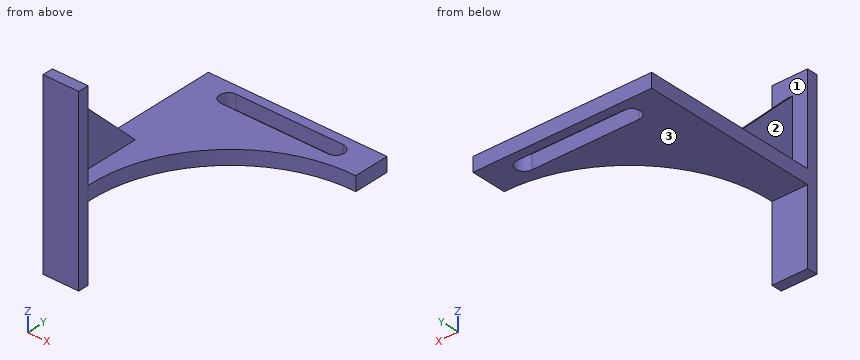
from build123d import *

# Parameters (mm, degrees)
SKETCH1_W           = 50
SKETCH1_H           = 15
BOSS_EXTRUDE1_DEPTH = 250
BOSS_EXTRUDE3_START = -135
BOSS_EXTRUDE3_DEPTH = 10
BOSS_EXTRUDE4_DEPTH = 3.75
CUT_EXTRUDE1_DEPTH  = 365.082751583


with BuildPart() as part:
    # Sketch1 → Boss-Extrude1 (new body)
    with BuildSketch(Plane.XY):
        Rectangle(SKETCH1_W, SKETCH1_H)
    extrude(amount=-BOSS_EXTRUDE1_DEPTH)

    # Sketch2 → Boss-Extrude3 (add, symmetric)
    with BuildSketch(Plane.XY.offset(BOSS_EXTRUDE3_START)):
        with BuildLine():
            Line((-25, 7.5), (-25, 257.5))
            Line((-25, 257.5), (225, 257.5))
            Line((225, 257.5), (225, 207.5))
            ThreePointArc((225, 207.5), (82.048365399, 150.451634601), (25, 7.5))
            Line((25, 7.5), (-25, 7.5))
        make_face()
    extrude(amount=BOSS_EXTRUDE3_DEPTH, both=True)

    # Sketch4 → Boss-Extrude4 (add, symmetric)
    with BuildSketch(Plane(origin=(0, 0, 0), x_dir=(0, 0, -1), z_dir=(1, 0, 0))):
        Polygon((25, 7.5), (125, 107.5), (125, 7.5), align=None)
    extrude(amount=BOSS_EXTRUDE4_DEPTH, both=True)

    # Sketch5 → Cut-Extrude1 (cut, through all)
    with BuildSketch(Plane.XY.offset(-125)):
        with BuildLine():
            Line((25, 244.5), (175, 244.5))
            ThreePointArc((175, 244.5), (187, 232.5), (175, 220.5))
            Line((175, 220.5), (25, 220.5))
            ThreePointArc((25, 220.5), (13, 232.5), (25, 244.5))
        make_face()
    extrude(amount=-CUT_EXTRUDE1_DEPTH, mode=Mode.SUBTRACT)


solid = part.part
Can you work these out from the model? Positions are in its coordinate system, mm. Face numbers are marked on the shaded views. A direction names the side the tool comes from. Give positions to 0.01 mm unless a question says otherwise; leave off trailing zeros. Write each loop counter-clockwise with the first axis right and the second up, starting at its lowest first coordinate (ties: lowest second). Pieces come first, ordered by that corner, then holes. Notation, with made-up numbers: (15, 62) -> (71, 62) arc R27 ccw to (71, 78) -> close; hole circle Ø9 at (-37, 45). An arc over 180 degrees is marked (long way). Answer as a JSON object with one key per item and string values. Group by question number.
Item 1: Suppose I cut it at D-D (y = 23). Please give me the cut outline in (x, z), plus the area to 3 significant figures.
Item 2: Please list where these lines run through material, in increasing order: line 1 (X direction, y = 26.5, z = -46); line 2 (Z direction, x = 130.5, y = 219.5); line 3 (Y direction, x = 20, z = -50.5). Write a range as [from, to].
Item 3: For the marked faces 1, 2 and 3, which set-ups out of +Z, -Z, +X, -X, +Y, -Y let a thin tool reach every point of the face, with its end or its side?
Item 4: Suppose I cut it at B-B (x = 83.5). Please give me the cut outline in (y, z).
Item 5: Suppose I cut it at C-C (z = -113.5). Please give me the cut outline in (x, y), plus the area to 3 significant figures.
Item 6: I'm going to push flat-ended pins straight in: P1, Ø4, axis at y = 26, z = -100.5, coming from the -X side; P2, Ø4, axis at x = 96.5, y = 201.5, coming from the -Z side; P3, Ø25, axis at x = -2, z = -213.5, coming from the +Y side. Where does each tip first touch, or does it pass through?
Item 7: Suppose I cut it at A-A (y = 232.5). Please give me the cut outline in (x, z).
Findings:
{
 "1": {"outline": "(-25, -145) -> (25.21, -145) -> (25.21, -125) -> (3.75, -125) -> (3.75, -40.5) -> (-3.75, -40.5) -> (-3.75, -125) -> (-25, -125) -> close", "area": "1,640 mm²"},
 "2": {"line 1": "x = [-3.75, 3.75]", "line 2": "z = [-145, -125]", "line 3": "y = [-7.5, 7.5]"},
 "3": {"face 1": "+Z, +Y", "face 2": "+Z, -X, +Y", "face 3": "-Z, +X, -X, +Y"},
 "4": {"outline": "(151.89, -145) -> (220.5, -145) -> (220.5, -125) -> (151.89, -125) -> close; (244.5, -145) -> (257.5, -145) -> (257.5, -125) -> (244.5, -125) -> close"},
 "5": {"outline": "(-25, -7.5) -> (25, -7.5) -> (25, 7.5) -> (3.75, 7.5) -> (3.75, 96) -> (-3.75, 96) -> (-3.75, 7.5) -> (-25, 7.5) -> close", "area": "1,410 mm²"},
 "6": {"P1": "stops at x = -3.75", "P2": "stops at z = -145", "P3": "stops at y = 7.5"},
 "7": {"outline": "(-25, -145) -> (13, -145) -> (13, -125) -> (-25, -125) -> close; (187, -145) -> (225, -145) -> (225, -125) -> (187, -125) -> close"}
}
